The listing builds one solid part. Answer for the finished solid, in the listing's coordinates (mm). Give positions to 0.01 mm unless a question says otherwise; leave off trailing zeros. Return JSON: item names as keys, results as strings.
from build123d import *

# Parameters (mm, degrees)
F2_DEPTH = 3
F4_COUNT = 6


with BuildPart() as f2:
    # F1 (on Top) → F2 (new body)
    with BuildSketch(Plane.XY):
        Polygon((-3.143853, 2.46645), (0, 0), (2.705809, 1.481498), (2.705809, 11.658775), (11.181849, 16.792152), (11.181849, 6.122341), (17.15089, 9.390539), (17.15089, 27.178286), (3.143853, 18.582864), (3.143853, 24.671286), (17.588934, 33.50547), (14.577311, 38.42988), (3.214115, 31.480487), (3.214115, 37.564415), (11.739274, 42.817172), (8.440727, 48.170671), (2.623938, 44.58667), (2.623938, 50.576929), (0, 50.576929), (-2.623938, 50.576929), (-2.623938, 44.58667), (-8.440727, 48.170671), (-11.739274, 42.817172), (-3.214115, 37.564415), (-3.214115, 31.480487), (-14.577311, 38.42988), (-17.588934, 33.50547), (-3.143853, 24.671286), align=None)
    extrude(amount=F2_DEPTH)


with BuildPart() as f4_1:
    # F4: instance of F2
    add(f2.part.rotate(Axis((0, 0, 4.922884), (0, 0, 1)), 1 * 360 / F4_COUNT))


with BuildPart() as f4_2:
    # F4: instance of F2
    add(f2.part.rotate(Axis((0, 0, 4.922884), (0, 0, 1)), 2 * 360 / F4_COUNT))


with BuildPart() as f4_3:
    # F4: instance of F2
    add(f2.part.rotate(Axis((0, 0, 4.922884), (0, 0, 1)), 3 * 360 / F4_COUNT))


with BuildPart() as f4_4:
    # F4: instance of F2
    add(f2.part.rotate(Axis((0, 0, 4.922884), (0, 0, 1)), 4 * 360 / F4_COUNT))


with BuildPart() as f4_5:
    # F4: instance of F2
    add(f2.part.rotate(Axis((0, 0, 4.922884), (0, 0, 1)), 5 * 360 / F4_COUNT))


with BuildPart() as f2_1:
    add(f2.part)

    # F5: union F4_5, F4_3, F4_1, F4_2, F4_4
    add(f4_5.part)
    add(f4_3.part)
    add(f4_1.part)
    add(f4_2.part)
    add(f4_4.part)


solid = f2_1.part
Item 1: Flat-ended cylindrical pins translate along their axes: P1, Ø0.9, axis at y = 21, z = 1, coming from the +X side; P2, Ø1.5, axis at y = -7.5, z = 2, coming from the -X side; P3, Ø1, axis at x = 22.5, z = 2.5, coming from the +Y side. Find the tip coordinate at first contact, or state that the pin passes through.
Answer below:
{"P1": "stops at x = 42.4", "P2": "stops at x = -40.28", "P3": "stops at y = 31.94"}
Item 2: Consider L1, parallel to Y at x = -38, z = 1; L2, parallel to Y at x = 21, z = 1.1; L3, parallel to Y at x = -23, z = 1.05. Determine where each line is inside the solid, lowest interval first.
Answer below:
{"L1": "y = -24.97 to -13.91, -7.99 to -1.87, 1.87 to 7.99, 13.91 to 24.97", "L2": "y = -31.97 to -8.49, -7.68 to 4.76, 8.49 to 31.97", "L3": "y = -31.91 to -9.58, -3.68 to 6.53, 9.58 to 31.91"}
Item 3: A cutting plane is placed at A-A on z = 0.55. Give the number of separate pieces and of enclosed holes in the cut face, then the cut area to 3 significant figures.
Answer below:
{"separate pieces": "1", "enclosed holes": "6", "area": "4,230 mm²"}
